The listing builds one solid part. Answer for the finished solid, in the listing's coordinates (mm). A direction names the side the tool comes from. Coordinates: 2 decimals unless noted, no trailing zeros. Write each loop counter-clockwise with the first axis right and the second up, starting at its lowest first coordinate (ties: lowest second). Pieces come first, ordered by that corner, then holes.
```python
from build123d import *

# Parameters (mm, degrees)
SKETCH3_OUTSIDE_W   = 25.668
SKETCH3_OUTSIDE_H   = 25.668
CUT_EXTRUDE1_DEPTH  = 47.788336733
CHAMFER1_SIZE       = 0.508
BOSS_EXTRUDE1_DEPTH = 15.6718
FILLET1_R           = 0.508


with BuildPart() as part:
    # Sketch2 → Revolve1 (revolve)
    with BuildSketch(Plane(origin=(0, 0, 0), x_dir=(0, 0, -1), z_dir=(1, 0, 0)), mode=Mode.PRIVATE) as revolve1_sk:
        Polygon((-22.8854, 6.35), (-22.8854, 0), (22.8854, 0), (22.8854, 4.7625), (15.748, 4.7625), (15.748, 6.862299966), (-20.6248, 6.862299966), (-20.6248, 5.8928), (-21.6154, 5.8928), (-21.6154, 6.35), align=None)
    revolve(revolve1_sk.sketch.rotate(Axis((0, 0, 6.497503614), (0, 0, -1)), 90), axis=Axis((0, 0, 6.497503614), (0, 0, -1)))

    # Sketch3 outside → Cut-Extrude1 (cut, through all)
    with BuildSketch(Plane.XY.offset(22.8854)):
        Rectangle(SKETCH3_OUTSIDE_W, SKETCH3_OUTSIDE_H)
        Polygon((1.509607841, -7.238192802), (7.023262765, -2.311737661), (5.513654923, 4.926455141), (-1.509607841, 7.238192802), (-7.023262765, 2.311737661), (-5.513654923, -4.926455141), align=None, mode=Mode.SUBTRACT)
    extrude(amount=-CUT_EXTRUDE1_DEPTH, mode=Mode.SUBTRACT)

    # Chamfer1
    chamfer1_edges = [part.edges().sort_by_distance(p)[0] for p in [
        (-6.35, 0, 22.8854),
        (-4.7625, 0, -22.8854),
    ]]
    chamfer(chamfer1_edges, length=CHAMFER1_SIZE)

    # Sketch4 → Boss-Extrude1 (add)
    with BuildSketch(Plane(origin=(0, 0, -15.748), x_dir=(-1, 0, 0), z_dir=(0, 0, -1))):
        Polygon((-1.509607841, -7.238192802), (5.513654923, -4.926455141), (7.023262765, 2.311737661), (1.509607841, 7.238192802), (-5.513654923, 4.926455141), (-7.023262765, -2.311737661), align=None)
    extrude(amount=-BOSS_EXTRUDE1_DEPTH)

    # Fillet1
    fillet1_edges = [part.edges().sort_by_distance(p)[0] for p in [
        (1.509607841, -7.238192802, -7.9121),
        (7.023262765, -2.311737661, -7.9121),
        (5.513654923, 4.926455141, -7.9121),
        (-1.509607841, 7.238192802, -7.9121),
        (-7.023262765, 2.311737661, -7.9121),
        (-5.513654923, -4.926455141, -7.9121),
    ]]
    fillet(fillet1_edges, radius=FILLET1_R)


solid = part.part
```
(1) Section B-B, the plane y = 0 is taken. Write down the section's boundary in (x, z).
(2) Each of these flat-tipped pins is pushed along its axis until it touches: pin 1 (8 mm diameter, centred on y = 1, z = 12, fed in from -X); pin 2 (1 mm diameter, centred on x = 6.5, y = -2, fed in from +Z); pin 3 (0.8 mm diameter, centred on x = -1.5, y = 6.5, fed in from +Z); pin 4 (8 mm diameter, centred on y = 2.5, z = 1.5, fed in from -X). Where does it stop, or does it pass through?
(3) Which of the six approach directions +Z, -Z, +X, -X, +Y, -Y give full straight-line access (tool end or side, diameter ignored) to faces 4 (the flat face through (-6.7, 2.2, -0.076)), 5 (the cylindrical face through (1.416, -6.715, 10.419)), 6 (the cylindrical face through (5.11, 4.58, 10.42)), 7 (the cylindrical face through (-5.11, -4.58, 10.42)), 8 (the flat face through (-2, 6, 20.625))?
(4) Section C-C, the plane z = 9 is taken. Write down the section's boundary in (x, y).
(5) Section A-A, the plane z = -10 is taken. Write down the section's boundary in (x, y).
(6) Section D-D, the plane z = -17.5 is taken. Write down the section's boundary in (x, y) (1 decimal).
(7) Find the intervals of material crossed by probe 1 along Z at (x, y) = (-5.5, -0.25); probe 2 along Z at (x, y) = (-2.5, 5.5); probe 3 along X at (y, z) = (-2, 19), in increasing order.
(8) For a pull along Z with two mould halves and no side action, classify faces 1 (the flat face through (-4.23, 4.81, 2.69)), 2 (the cylindrical face through (-0.767, -5.843, 21.127)), 3 (the flat face through (5.3, 4.6, -0.076)) as pulls with the +Z half, pulls with the -Z half, needs draft (parallel to the pull), parting line crosses it, or undercut.
Solution:
1. outline: (-6.54, -15.75) - (-4.76, -15.75) - (-4.76, -22.38) - (-4.25, -22.89) - (4.25, -22.89) - (4.76, -22.38) - (4.76, -15.75) - (6.54, -15.75) - (6.54, 20.62) - (5.89, 20.62) - (5.89, 21.62) - (6.35, 21.62) - (6.35, 22.38) - (5.84, 22.89) - (-5.84, 22.89) - (-6.35, 22.38) - (-6.35, 21.62) - (-5.89, 21.62) - (-5.89, 20.62) - (-6.54, 20.62) - close
2. pin 1: stops at x = -6.77
2. pin 2: stops at z = 22.43
2. pin 3: stops at z = 22.46
2. pin 4: stops at x = -6.97
3. face 4: +Z, -X, +Y
3. face 5: +Z, +X, -Y
3. face 6: +Z, +X, +Y
3. face 7: +Z, -X, -Y
3. face 8: none
4. outline: (-6.77, 1.11) - (-5.76, -3.72) arc R6.86 ccw to (-4.35, -5.31) - (0.34, -6.85) arc R6.86 ccw to (2.43, -6.42) - (6.11, -3.13) arc R6.86 ccw to (6.77, -1.11) - (5.76, 3.72) arc R6.86 ccw to (4.35, 5.31) - (-0.34, 6.85) arc R6.86 ccw to (-2.43, 6.42) - (-6.11, 3.13) arc R6.86 ccw to start
5. outline: (-6.96, 2.02) - (-5.57, -4.64) arc R0.51 ccw to (-5.24, -5.02) - (1.23, -7.15) arc R0.51 ccw to (1.73, -7.04) - (6.8, -2.51) arc R0.51 ccw to (6.96, -2.02) - (5.57, 4.64) arc R0.51 ccw to (5.24, 5.02) - (-1.23, 7.15) arc R0.51 ccw to (-1.73, 7.04) - (-6.8, 2.51) arc R0.51 ccw to start
6. outline: circle Ø9.5 at (0, 0)
7. probe 1: z = -15.75 to 22.89
7. probe 2: z = -15.75 to 20.62, 21.62 to 22.69
7. probe 3: x = -6.12 to 6.56
8. face 1: needs draft
8. face 2: undercut
8. face 3: pulls with the +Z half
